The listing builds one solid part. Answer for the finished solid, in the listing's coordinates (mm). A direction names the side the tool comes from. Give positions to 0.01 mm unless a question says otherwise; leave off trailing zeros. Write each loop counter-clockwise with the first axis right and the second up, starting at its lowest first coordinate (ties: lowest second). Pieces come first, ordered by that corner, then holes. Notation, with made-up numbers: (-26, -17) - (23, -17) arc R27 ccw to (23, 6) - close; hole circle Ø2 at (15.25, 82). An arc over 180 degrees is marked (long way). Write each question's results on one line, items separated by ' | '. Start each with the question number.
Q1. A flat-ended cylindrical pin translates along its axis: pin 1 Ø0.8 at (y, z) = (-1.5, 0.5) entering from +X. Find the tip coordinate at first contact, or state that the pin passes through.
Q2. Section C-C (z = 0) is taken. Determine the outline of the cut face in (x, y), plus the area to 3 significant figures.
Q3. For a pull along Y with two mould halves and no side action, classify faces 4 (the face through (-2.059, -1, 0)), 5 (the face through (7.463, -1.294, 3.492)), 6 (the face through (3.3, 0, 2.3)) as pulls with the +Y half, pulls with the -Y half, needs draft (parallel to the pull), parting line crosses it, or undercut.
Q4. Section A-A (x = 3) is taken. Determine the outline of the cut face in (y, z).
Q5. Find the intervals of material crossed by probe 1 along Z at (x, y) = (0.75, -0.7); probe 2 along X at (y, z) = (-1.05, -4.5); probe 3 along X at (y, z) = (-1.2, 3.25), in increasing order.
Q6. Section B-B (y = -1.25) is taken. Determine the outline of the cut face in (x, z).
Q7. For faces 1 (the face through (7.463, -1.294, -3.449)), 2 (the face through (-5.291, -1.033, -0.976)), 3 (the face through (4, -1, 1.941)), determine the directions among +Z, -Z, +X, -X, +Y, -Y from which every point of the face is accessible in a straight line to the end or side of a thin tool.
```python
from build123d import *

# Parameters (mm, degrees)
F2_W     = 2
F2_H     = 3.0588235933
F2_H_2   = 3.8823528133
F3_DEPTH = 2.5
F5_D     = 2
F6_R     = 1
F7_DEPTH = 2.5


with BuildPart() as f3:
    # F2 (on Front) → F3 (new body)
    with BuildSketch(Plane.XZ):
        with Locations((-3.058823533, 3.4705882033)):
            Rectangle(F2_W, F2_H)
        Polygon((-0.058823533, 5), (-2.058823533, 5), (-2.058823533, 1.9411764067), (10.941176467, 1.9411764067), (10.941176467, 5), align=None)
        with Locations((-3.058823533, 0)):
            Rectangle(F2_W, F2_H_2)
        with Locations((-3.058823533, -3.4705882033)):
            Rectangle(F2_W, F2_H)
        Polygon((10.941176467, -1.9411764067), (-2.058823533, -1.9411764067), (-2.058823533, -5), (-0.058823533, -5), (10.941176467, -5), align=None)
    extrude(amount=F3_DEPTH)

    # F5 (through all)
    with Locations(Plane(origin=(0, 0, -5), x_dir=(1, 0, 0), z_dir=(0, 0, -1))):
        with Locations((6.4643374644, 1.25)):
            Hole(F5_D / 2)

    # F6 (on face) → F7 (join)
    with BuildSketch(Plane(origin=(-4.058823533, 0, 0), x_dir=(0, -1, 0), z_dir=(-1, 0, 0))):
        with Locations((1.25, 0)):
            Circle(F6_R)
    extrude(amount=F7_DEPTH)


solid = f3.part
```
Answers below:
1) pin 1: stops at x = -2.06
2) outline: (-6.56, -2.25) - (-4.06, -2.25) - (-4.06, -2.5) - (-2.06, -2.5) - (-2.06, 0) - (-4.06, 0) - (-4.06, -0.25) - (-6.56, -0.25) - close | area: 10.0 mm2
3) face 4: needs draft | face 5: undercut | face 6: pulls with the +Y half
4) outline: (-2.5, -5) - (0, -5) - (0, -1.94) - (-2.5, -1.94) - close; (-2.5, 1.94) - (0, 1.94) - (0, 5) - (-2.5, 5) - close
5) probe 1: z = -5 to -1.94, 1.94 to 5 | probe 2: x = -4.06 to 5.48, 7.44 to 10.94 | probe 3: x = -4.06 to 5.47, 7.46 to 10.94
6) outline: (-6.56, -1) - (-4.06, -1) - (-4.06, -5) - (5.46, -5) - (5.46, -1.94) - (-2.06, -1.94) - (-2.06, 1.94) - (5.46, 1.94) - (5.46, 5) - (-4.06, 5) - (-4.06, 1) - (-6.56, 1) - close; (7.46, -5) - (10.94, -5) - (10.94, -1.94) - (7.46, -1.94) - close; (7.46, 1.94) - (10.94, 1.94) - (10.94, 5) - (7.46, 5) - close
7) face 1: +Z, -Z | face 2: -X | face 3: +X, +Y, -Y
